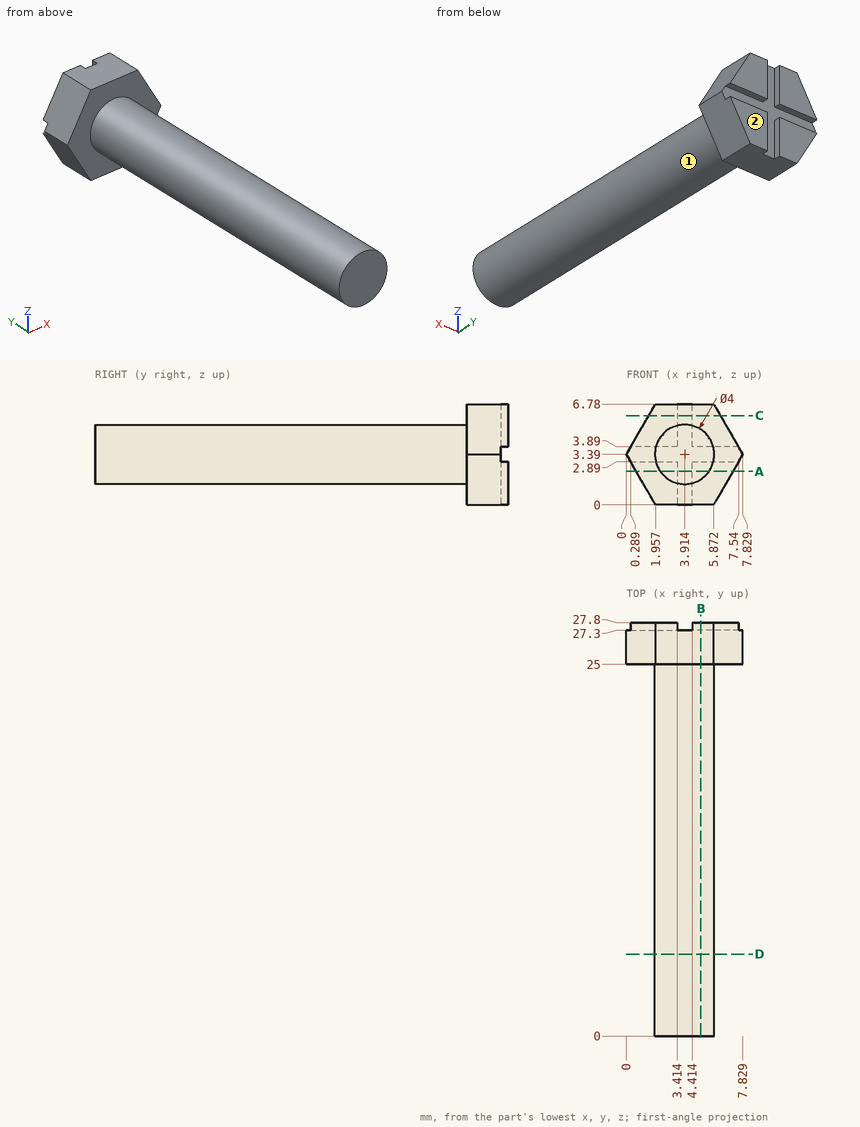
Job drawing, mm, ordinate dimensions from the low corner. One solid piece. A direction names the side the tool comes from. Give positions to 0.01 mm unless a question says otherwise; leave off trailing zeros. Write each loop counter-clockwise with the first axis right and the second up, starting at its lowest first coordinate (ties: lowest second). Pieces come first, ordered by that corner, then holes. Notation, with made-up numbers: M 68,17 L 92,17 A19 cw 92,33 Z; hole C -25,-3 d10. An arc over 180 degrees is marked long. Put each result on its own line as item: value. Start each with the question number.
(1) Probe L1, parallel to X at y = 21.5, z = 3.25; L2, parallel to Y at x = 4.75, z = 5.25; L3, parallel to Y at x = 4.25, z = 2. List the from-to ranges inside material, lowest first.
(2) Band-saw the part on D-D, the plane y = 5.5. Write the cut outline in (x, z) (1 decimal).
(3) Band-saw the part on A-A, the plane z = 2.25. Write the cut outline in (x, y) (1 decimal).
(4) Band-saw the part on C-C, the plane z = 6. Write the cut outline in (x, y) (1 decimal), and give its area (3 significant figures).
(5) Which spindle directions (+Z, -Z, +X, -X, +Y, -Y) get a long thin tool onto all of the face, cutting with end or side? Do the marked faces 1 and 2. Say none if no direction does.
(6) Band-saw the part on B-B, the plane x = 5. Write the cut outline in (y, z).
(7) Flat gauge pins, fed straight in: pin 1 Ø1.5 at (x, y) = (1.5, 11) entering from -Z; pin 2 Ø4 at (x, y) = (2.5, 6.5) entering from +Z; pin 3 Ø2 at (y, z) = (19.5, 2.5) entering from -X. Where does each tip first touch, or does it go through?
Response values:
1. L1: x = 1.92 to 5.91
1. L2: y = 25 to 27.8
1. L3: y = 0 to 27.3
2. outline: C 3.9,3.4 d4
3. outline: M 0.7,25 L 2.3,25 L 2.3,0 L 5.6,0 L 5.6,25 L 7.2,25 L 7.2,27.8 L 4.4,27.8 L 4.4,27.3 L 3.4,27.3 L 3.4,27.8 L 0.7,27.8 Z
4. outline: M 1.5,25 L 6.3,25 L 6.3,27.8 L 4.4,27.8 L 4.4,27.3 L 3.4,27.3 L 3.4,27.8 L 1.5,27.8 Z
4. area: 13.0 mm2
5. face 1: -Y
5. face 2: +Z, -Z, +X, -X, +Y
6. outline: M 0,1.71 L 25,1.71 L 25,0 L 27.8,0 L 27.8,2.89 L 27.3,2.89 L 27.3,3.89 L 27.8,3.89 L 27.8,6.78 L 25,6.78 L 25,5.07 L 0,5.07 Z
7. pin 1: stops at z = 2.28
7. pin 2: stops at z = 5.39
7. pin 3: stops at x = 1.91
